```python
from build123d import *

# Parameters (mm, degrees)
EXTRUDE_1_DEPTH     = 9.6
SKETCH_2_R          = 2.4
EXTRUDE_2_DEPTH     = 1.7
SKETCH_3_R          = 2.5
CUT_EXTRUDE_1_DEPTH = 1.8


with BuildPart() as part:
    # Эскиз1 → Бобышка-Вытянуть1 (new body)
    with BuildSketch(Plane.XY):
        Polygon((7.9, 7.9), (-7.9, 7.9), (-7.9, 0), (0, 0), (0, -7.9), (7.9, -7.9), align=None)
    extrude(amount=EXTRUDE_1_DEPTH)

    # Эскиз2 → Бобышка-Вытянуть2 (add)
    with BuildSketch(Plane.XY.offset(9.6)):
        with Locations(Location((-4, 4, 0), (0, 0, 180))):
            Circle(SKETCH_2_R)
        with Locations(Location((4, 4, 0), (0, 0, 180))):
            Circle(SKETCH_2_R)
        with Locations(Location((4, -4, 0), (0, 0, 180))):
            Circle(SKETCH_2_R)
    extrude(amount=EXTRUDE_2_DEPTH)

    # Эскиз3 → Вырез-Вытянуть1 (cut)
    with BuildSketch(Plane(origin=(0, 0, 0), x_dir=(-1, 0, 0), z_dir=(0, 0, -1))):
        with Locations((4, 4)):
            Circle(SKETCH_3_R)
        with Locations((-4, 4)):
            Circle(SKETCH_3_R)
        with Locations((-4, -4)):
            Circle(SKETCH_3_R)
    extrude(amount=-CUT_EXTRUDE_1_DEPTH, mode=Mode.SUBTRACT)


solid = part.part
```
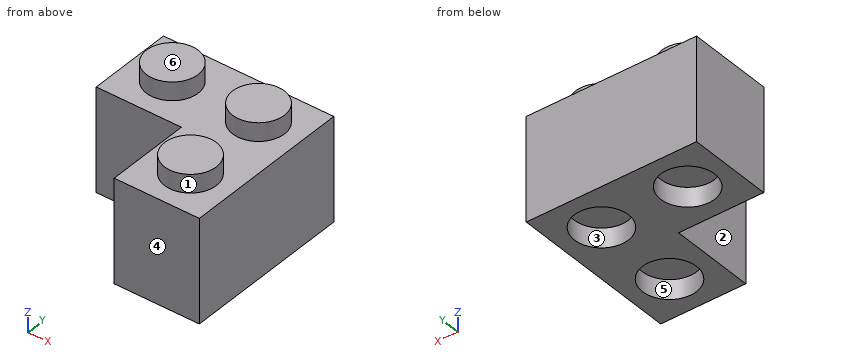
Source: CAD feature listing. Evaluate the final solid. Frame: model axes, mm. Face numbers are marked on the shaded views. A direction names the side the tool comes from. Coordinates: 2 decimals unless noted, no trailing zeros. Write each loop counter-clockwise with the first axis right and the second up, starting at its lowest first coordinate (ties: lowest second). Pieces come first, ordered by that corner, then holes. Notation, with made-up numbers: (-1.5, 63) -> (42.5, 63) arc R19 ccw to (42.5, 85) -> close; hole circle Ø10 at (12, 79.5). An arc over 180 degrees is marked (long way). Return JSON: item names as keys, results as strings. Group by question number.
1) Section query A-A, the plane y = 4. Return loops of the section in (x, z).
2) Mould query, pull axis Y, two halves, no side actions, for the marked faces 4, 5 and 6. Classes: +Y half, -Y half, draft (parallel to the pull), parting line (faces both ways), or undercut.
3) Contact query for flat-ended pins moving along their axis: P1, Ø2.5, axis at x = 3.5, y = -3, coming from the -Z side; P2, Ø1.5, axis at x = -2, y = 0.5, coming from the +Z side; P3, Ø4, axis at y = -5, z = 7, coming from the -X side. Output: stop coordinate, or through.
4) Set-up query: the marked faces 1, 2 and 3. Return all of +Z, -Z, +X, -X, +Y, -Y with unobstructed straight access to the full face (end or side cutting, diameter ignored); none if empty.
5) Section query C-C, the plane z = 2.5. Return loops of the section in (x, y), plus the area to 3 significant figures.
6) Section query B-B, the plane x = -4. Return loops of the section in (y, z), plus the area to 3 significant figures.
7) Ray query, line 1 along Y through (x, z) = (4, 1.05); line 2 along Y through (x, z) = (3, 1.75); line 3 along Y through (x, z) = (-4, 1.4). Return the intervals inside material, ascending.
From the geometry:
{
 "1": {"outline": "(-7.9, 0) -> (-6.5, 0) -> (-6.5, 1.8) -> (-1.5, 1.8) -> (-1.5, 0) -> (1.5, 0) -> (1.5, 1.8) -> (6.5, 1.8) -> (6.5, 0) -> (7.9, 0) -> (7.9, 9.6) -> (6.4, 9.6) -> (6.4, 11.3) -> (1.6, 11.3) -> (1.6, 9.6) -> (-1.6, 9.6) -> (-1.6, 11.3) -> (-6.4, 11.3) -> (-6.4, 9.6) -> (-7.9, 9.6) -> close"},
 "2": {"face 4": "-Y half", "face 5": "undercut", "face 6": "draft"},
 "3": {"P1": "z = 1.8", "P2": "z = 9.6", "P3": "x = 0"},
 "4": {"face 1": "+Z", "face 2": "+Z, -Z, -X, -Y", "face 3": "-Z"},
 "5": {"outline": "(-7.9, 0) -> (0, 0) -> (0, -7.9) -> (7.9, -7.9) -> (7.9, 7.9) -> (-7.9, 7.9) -> close", "area": "187 mm²"},
 "6": {"outline": "(0, 0) -> (1.5, 0) -> (1.5, 1.8) -> (6.5, 1.8) -> (6.5, 0) -> (7.9, 0) -> (7.9, 9.6) -> (6.4, 9.6) -> (6.4, 11.3) -> (1.6, 11.3) -> (1.6, 9.6) -> (0, 9.6) -> close", "area": "75.0 mm²"},
 "7": {"line 1": "-7.9 to -6.5, -1.5 to 1.5, 6.5 to 7.9", "line 2": "-7.9 to -6.29, -1.71 to 1.71, 6.29 to 7.9", "line 3": "0 to 1.5, 6.5 to 7.9"}
}
